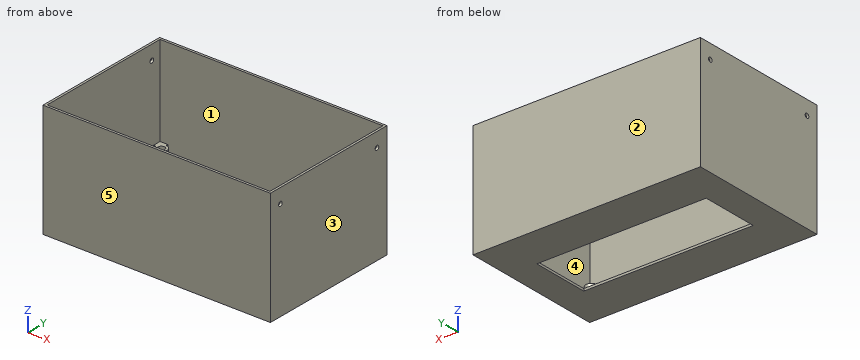
```python
from build123d import *

# Parameters (mm, degrees)
SKETCH_1_W               = 102
SKETCH_1_H               = 64
SKETCH_1_W_2             = 100
SKETCH_1_H_2             = 62
EXTRUDE_1_DEPTH          = 50
SKETCH_1_3_R             = 1.5
EXTRUDE_2_DEPTH          = 9.72
SKETCH_4_W               = 102
SKETCH_4_H               = 1
EXTRUDE_3_DEPTH          = 64
SKETCH_1_5_W             = 76
SKETCH_1_5_H             = 25.8
CUT_EXTRUDE_1_DEPTH      = 1
CUT_EXTRUDE_2_DEPTH      = 102
CUT_EXTRUDE_2_DEPTH_BACK = 1
SKETCH_5_R               = 1


with BuildPart() as part:
    # Sketch 1 → Extrude 1 (new body)
    with BuildSketch(Plane.XY):
        with Locations((53, 34)):
            Rectangle(SKETCH_1_W, SKETCH_1_H)
        with Locations((53, 34)):
            Rectangle(SKETCH_1_W_2, SKETCH_1_H_2, mode=Mode.SUBTRACT)
    extrude(amount=EXTRUDE_1_DEPTH)

    # Sketch 1_3 → Extrude 2 (add)
    # profile 1 of 4: a face of its own
    with BuildSketch(Plane.XY):
        with BuildLine():
            Line((6.5, 65), (3, 65))
            Line((3, 65), (3, 61.5))
            Line((3, 61.5), (4, 61.5))
            ThreePointArc((4, 61.5), (8.267766953, 59.732233047), (6.5, 64))
            Line((6.5, 64), (6.5, 65))
        make_face()
        with Locations((6.5, 61.5)):
            Circle(SKETCH_1_3_R, mode=Mode.SUBTRACT)
    # profile 2 of 4: a face of its own
    with BuildSketch(Plane.XY):
        with BuildLine():
            Line((103, 65), (99.5, 65))
            Line((99.5, 65), (99.5, 64))
            ThreePointArc((99.5, 64), (97.732233047, 59.732233047), (102, 61.5))
            Line((102, 61.5), (103, 61.5))
            Line((103, 61.5), (103, 65))
        make_face()
        with Locations((99.5, 61.5)):
            Circle(SKETCH_1_3_R, mode=Mode.SUBTRACT)
    # profile 3 of 4: a face of its own
    with BuildSketch(Plane.XY):
        with BuildLine():
            Line((103, 3), (103, 6.5))
            Line((103, 6.5), (102, 6.5))
            ThreePointArc((102, 6.5), (97.732233047, 8.267766953), (99.5, 4))
            Line((99.5, 4), (99.5, 3))
            Line((99.5, 3), (103, 3))
        make_face()
        with Locations((99.5, 6.5)):
            Circle(SKETCH_1_3_R, mode=Mode.SUBTRACT)
    # profile 4 of 4: a face of its own
    with BuildSketch(Plane.XY):
        with BuildLine():
            Line((4, 6.5), (3, 6.5))
            Line((3, 6.5), (3, 3))
            Line((3, 3), (6.5, 3))
            Line((6.5, 3), (6.5, 4))
            ThreePointArc((6.5, 4), (8.267766953, 8.267766953), (4, 6.5))
        make_face()
        with Locations((6.5, 6.5)):
            Circle(SKETCH_1_3_R, mode=Mode.SUBTRACT)
    extrude(amount=EXTRUDE_2_DEPTH)

    # Sketch 4 → Extrude 3 (add)
    with BuildSketch(Plane(origin=(0, 66, 0), x_dir=(1, 0, 0), z_dir=(0, 1, 0))):
        with Locations((53, 0.5)):
            Rectangle(SKETCH_4_W, SKETCH_4_H)
    extrude(amount=-EXTRUDE_3_DEPTH)

    # Sketch 1_5 → Cut-Extrude 1 (cut)
    with BuildSketch(Plane.XY):
        with Locations((53, 34)):
            Rectangle(SKETCH_1_5_W, SKETCH_1_5_H)
    extrude(amount=-CUT_EXTRUDE_1_DEPTH, mode=Mode.SUBTRACT)

    # Sketch 5 → Cut-Extrude 2 (cut, two sides: drawn at the far end of the back side and taken through both)
    with BuildSketch(Plane.ZY.offset(-103).offset(-CUT_EXTRUDE_2_DEPTH_BACK)):
        with Locations(Location((43.5, 7.5, 0), (0, 0, 90))):
            Circle(SKETCH_5_R)
        with Locations(Location((43.5, 60.5, 0), (0, 0, 90))):
            Circle(SKETCH_5_R)
    extrude(amount=CUT_EXTRUDE_2_DEPTH + CUT_EXTRUDE_2_DEPTH_BACK, mode=Mode.SUBTRACT)


solid = part.part
```
Model file for the job. Use its own axes, mm. Face numbers are marked on the shaded views. A direction names the side the tool comes from. Coordinates: 2 decimals unless noted, no trailing zeros. Order: outer loops, then holes, each group sorted by start corner. A loop starts at its lowest first (then second) coordinate and runs counter-clockwise, first axis right, second up. Notation, with made-up numbers: (35, 63) -> (71, 63) arc R24 cw to (71, 82) -> close; hole circle Ø3 at (-27, 64.5). An arc over 180 degrees is marked (long way). Return JSON: item names as keys, results as strings.
Item 1: Mould opens along Y. For the marked faces 1, 2 and 3 say: pulls with the +Y half, pulls with the -Y half, needs draft (parallel to the pull), parting line crosses it, or undercut.
Model answer:
{"face 1": "undercut", "face 2": "pulls with the +Y half", "face 3": "needs draft"}
Item 2: Slice it at C-C (y = 17). Write the cut outline in (x, z).
Model answer:
{"outline": "(2, -1) -> (104, -1) -> (104, 50) -> (103, 50) -> (103, 0) -> (3, 0) -> (3, 50) -> (2, 50) -> close"}
Item 3: Slice it at B-B (x = 83). Write the cut outline in (y, z), then the cut area to 3 significant figures.
Model answer:
{"outline": "(2, -1) -> (21.1, -1) -> (21.1, 0) -> (3, 0) -> (3, 50) -> (2, 50) -> close; (46.9, -1) -> (66, -1) -> (66, 50) -> (65, 50) -> (65, 0) -> (46.9, 0) -> close", "area": "138 mm²"}
Item 4: Pin check, flat tips, straight feed: P1, Ø8, axis at x = 71, y = 44, coming from the -Z side; P2, Ø3.5, axis at x = 6.5, y = 7, coming from the +Z side. Stop position of each tip, or through.
Model answer:
{"P1": "stops at z = -1", "P2": "stops at z = 9.72"}
Item 5: Wall check: line 1 along Y through (x, z) = (2.2, 43.5); line 2 along Y through (x, z) = (8.5, 9); line 3 along X through (y, z) = (21.5, 45). Give the ranges that are in metal, low to high. Write a range as from..to.
Model answer:
{"line 1": "y = 2..6.5, 8.5..59.5, 61.5..66", "line 2": "y = 2..3, 5..8, 60..63, 65..66", "line 3": "x = 2..3, 103..104"}
Item 6: 3-axis set-ups, long thin cutter, end or side, ignore diameter. For the marked faces 4 and 5: which of +Z, -Z, +X, -X, +Y, -Y reach the whole face in a straight line?
Model answer:
{"face 4": "+Z", "face 5": "+Z, -Z, +X, -X, -Y"}
Item 7: Slice it at A-A (z = 28.5). Write the cut outline in (x, y), then the cut area to 3 significant figures.
Model answer:
{"outline": "(2, 2) -> (104, 2) -> (104, 66) -> (2, 66) -> close; hole (3, 3) -> (103, 3) -> (103, 65) -> (3, 65) -> close", "area": "328 mm²"}
